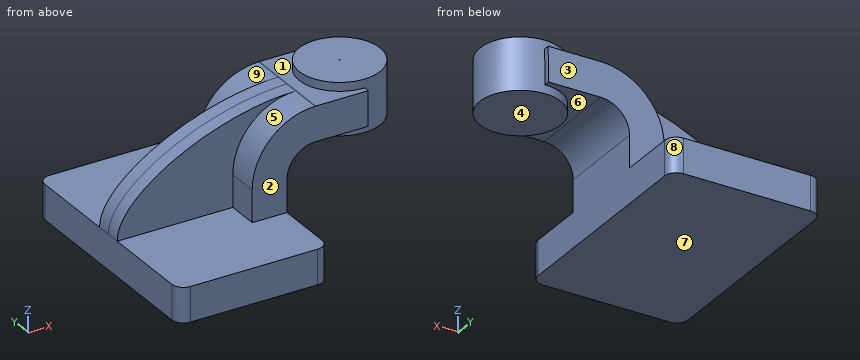
from build123d import *

# Parameters (mm, degrees)
F1_DEPTH = 63.5
F2_DEPTH = 25.4
F3_DEPTH = 7.9375
F5_R     = 6.35


with BuildPart() as f1:
    # F0 (on Front) → F1 (new body, symmetric)
    with BuildSketch(Plane.XZ):
        Polygon((-41.275, 9.525), (-41.275, -9.525), (41.275, -9.525), (41.275, 9.525), (22.225, 9.525), align=None)
    extrude(amount=F1_DEPTH, both=True)

    # F0 (on Front) → F2 (join, symmetric)
    with BuildSketch(Plane.XZ):
        with BuildLine():
            Line((22.225, 9.525), (41.275, 9.525))
            Line((41.275, 9.525), (41.275, 27.0002))
            ThreePointArc((41.275, 27.0002), (45.92468, 38.22552), (57.15, 42.8752))
            Line((57.15, 42.8752), (57.15, 61.9252))
            add(Edge.make_bspline(
                [(56.711113, 61.922442), (56.857474, 61.92365), (57.00377, 61.92457), (57.15, 61.9252)],
                knots=[111.150721, 111.150721, 111.150721, 111.150721, 111.504536, 111.504536, 111.504536, 111.504536], degree=3))
            ThreePointArc((56.711113, 61.922442), (32.29961, 51.540244), (22.225, 27.0002))
            Line((22.225, 27.0002), (22.225, 9.525))
        make_face()
        Polygon((85.957468, 61.9252), (57.15, 61.9252), (57.15, 42.8752), (85.725, 42.8752), align=None)
    extrude(amount=F2_DEPTH, both=True)

    # F0 (on Front) → F3 (join, symmetric)
    with BuildSketch(Plane.XZ):
        with BuildLine():
            add(Edge.make_bspline(
                [(-41.275, 9.525), (-41.625955, 32.723309), (10.731886, 61.543013), (56.711113, 61.922442)],
                knots=[0, 0, 0, 0, 111.150721, 111.150721, 111.150721, 111.150721], degree=3))
            Line((-41.275, 9.525), (22.225, 9.525))
            Line((22.225, 9.525), (22.225, 27.0002))
            ThreePointArc((22.225, 27.0002), (32.29961, 51.540244), (56.711113, 61.922442))
        make_face()
    extrude(amount=F3_DEPTH, both=True)

    # F0 (on Front) → F4 (revolve)
    with BuildSketch(Plane.XZ):
        Polygon((85.957468, 66.675), (85.957468, 61.9252), (85.725, 42.8752), (85.725, 38.1), (107.95, 38.1), (107.95, 66.675), align=None)
    revolve(axis=Axis((85.725, 0, 40.4876), (0, 0, 1)))

    # F5
    f5_edges = [f1.edges().sort_by_distance(p)[0] for p in [
        (-41.275, -63.5, 0),
        (41.275, -63.5, 0),
        (41.275, 63.5, 0),
        (-41.275, 63.5, 0),
    ]]
    fillet(f5_edges, radius=F5_R)


solid = f1.part
For this review, take the finished solid that the model builds, in its own axes (mm). Face numbers are marked on the shaded views. A direction names the side the tool comes from. Give positions to 0.01 mm unless a question says otherwise; leave off trailing zeros. Order: outer loops, then holes, each group sorted by start corner. A loop starts at its lowest first (then second) coordinate and runs counter-clockwise, first axis right, second up. Notation, with made-up numbers: (-11, 26.5) -> (46, 26.5) arc R35 cw to (46, 65.5) -> close; hole circle Ø11 at (69, 34). An arc over 180 degrees is marked (long way). Write item = value, one per line.
1) We need section A-A, the plane z = 0. Give the boundary of the cut face in (x, y) (3 decimals).
Findings:
outline = (-41.275, -57.15) arc R6.35 ccw to (-34.925, -63.5) -> (34.925, -63.5) arc R6.35 ccw to (41.275, -57.15) -> (41.275, 57.15) arc R6.35 ccw to (34.925, 63.5) -> (-34.925, 63.5) arc R6.35 ccw to (-41.275, 57.15) -> close
2) To check wall thickness, follow L1, parallel to Y at x = 50.5, z = 45; L2, parallel to Y at x = -1.5, z = 38.5; L3, parallel to Z at x = -27, y = 25 (3 decimals). State the ranges of each line that lie inside material, in increasing order. Write a range as from..to.
Findings:
L1 = -25.4..25.4
L2 = -7.94..7.94
L3 = -9.525..9.525
3) We need section B-B, the plane x = 74. Give the boundary of the cut face in (y, z) (3 decimals).
Findings:
outline = (-25.4, 42.875) -> (-18.881, 42.875) -> (-18.881, 38.1) -> (18.881, 38.1) -> (18.881, 42.875) -> (25.4, 42.875) -> (25.4, 61.925) -> (18.881, 61.925) -> (18.881, 66.675) -> (-18.881, 66.675) -> (-18.881, 61.925) -> (-25.4, 61.925) -> close
4) We need section C-C, the plane y = 29.5. Give the boundary of the cut face in (x, z) (3 decimals), and give its area (3 significant figures).
Findings:
outline = (-41.275, -9.525) -> (41.275, -9.525) -> (41.275, 9.525) -> (-41.275, 9.525) -> close
area = 1,570 mm^2
5) For the marked faces 1, 2, 3, 4 and 5, list the 3-axis set-ups (+Z, -Z, +X, -X, +Y, -Y) from which the entire face can be reached by the end or side of a thin tool; tool diameter is ignored.
Findings:
face_1 = +Z, -X
face_2 = +Z, +X, -X, -Y
face_3 = +Z, +X, -X, +Y
face_4 = -Z, +X, +Y, -Y
face_5 = +Z, -X, -Y
6) Draft analysis for pull direction X (two halves, no side actions). For the marked faces 6, 7, 8 and 9, state which applies: pulls with the +X half, pulls with the -X half, needs draft (parallel to the pull), parting line crosses it, or undercut.
Findings:
face_6 = undercut
face_7 = needs draft
face_8 = pulls with the +X half
face_9 = pulls with the -X half
7) Insertion check: pin 1 (5 mm diameter, centred on y = -1, z = 33, fed in from +X); pin 2 (1.5 mm diameter, centred on x = 43, z = 45.5, fed in from +Y); pin 3 (3 mm diameter, centred on y = 18.5, z = 0, fed in from +X) (3 decimals); pin 4 (10 mm diameter, centred on x = 89.5, y = -29.5, fed in from +Z). Each pin has a flat end and moves straight along its axis. Give the tip position at first contact, or say it passes through.
Findings:
pin_1 = 43.74
pin_2 = 25.4
pin_3 = 41.275
pin_4 = through
